from build123d import *

# Parameters (mm, degrees)
F0_R     = 160
F0_R_2   = 4.5
F0_R_3   = 4
F0_R_4   = 3.5
F0_R_5   = 125
F1_DEPTH = 5


with BuildPart() as f1:
    # F0 (on Top) → F1 (new body)
    with BuildSketch(Plane.XY):
        Circle(F0_R)
        with Locations((-89.58033, -123.296747)):
            Circle(F0_R_2, mode=Mode.SUBTRACT)
        with Locations((-123.296747, -89.58033)):
            Circle(F0_R_2, mode=Mode.SUBTRACT)
        with Locations((-106.988743, -92.985752)):
            Circle(F0_R_3, mode=Mode.SUBTRACT)
        with Locations((-91.955953, -96.538456)):
            Circle(F0_R_4, mode=Mode.SUBTRACT)
        with Locations((-47.095167, -144.944019)):
            Circle(F0_R_2, mode=Mode.SUBTRACT)
        with Locations((-73.121028, -121.182326)):
            Circle(F0_R_3, mode=Mode.SUBTRACT)
        with Locations((-32.197696, -137.533162)):
            Circle(F0_R_3, mode=Mode.SUBTRACT)
        with Locations((-17.947687, -131.571308)):
            Circle(F0_R_4, mode=Mode.SUBTRACT)
        with Locations((-57.726149, -119.915761)):
            Circle(F0_R_4, mode=Mode.SUBTRACT)
        with Locations((-144.944019, -47.095167)):
            Circle(F0_R_2, mode=Mode.SUBTRACT)
        with Locations((-130.485633, -55.703517)):
            Circle(F0_R_3, mode=Mode.SUBTRACT)
        with Locations((-117.286447, -63.727727)):
            Circle(F0_R_4, mode=Mode.SUBTRACT)
        with Locations((-131.238105, -24.695316)):
            Circle(F0_R_4, mode=Mode.SUBTRACT)
        with Locations((-141.31166, -12.985067)):
            Circle(F0_R_3, mode=Mode.SUBTRACT)
        with Locations((0, -152.403161)):
            Circle(F0_R_2, mode=Mode.SUBTRACT)
        with Locations((11.775392, -140.437726)):
            Circle(F0_R_3, mode=Mode.SUBTRACT)
        with Locations((23.485642, -130.364171)):
            Circle(F0_R_4, mode=Mode.SUBTRACT)
        with Locations((47.095167, -144.944019)):
            Circle(F0_R_2, mode=Mode.SUBTRACT)
        with Locations((54.493843, -129.611699)):
            Circle(F0_R_3, mode=Mode.SUBTRACT)
        with Locations((62.518052, -116.412512)):
            Circle(F0_R_4, mode=Mode.SUBTRACT)
        with Locations((89.58033, -123.296747)):
            Circle(F0_R_2, mode=Mode.SUBTRACT)
        with Locations((91.776078, -106.114808)):
            Circle(F0_R_3, mode=Mode.SUBTRACT)
        with Locations((95.328782, -91.082019)):
            Circle(F0_R_4, mode=Mode.SUBTRACT)
        with Locations((123.296747, -89.58033)):
            Circle(F0_R_2, mode=Mode.SUBTRACT)
        with Locations((119.972651, -72.247093)):
            Circle(F0_R_3, mode=Mode.SUBTRACT)
        with Locations((118.706086, -56.852215)):
            Circle(F0_R_4, mode=Mode.SUBTRACT)
        with Locations((144.944019, -47.095167)):
            Circle(F0_R_2, mode=Mode.SUBTRACT)
        with Locations((136.323487, -31.323761)):
            Circle(F0_R_3, mode=Mode.SUBTRACT)
        with Locations((130.361633, -17.073752)):
            Circle(F0_R_4, mode=Mode.SUBTRACT)
        with Locations((-152.403161, 0)):
            Circle(F0_R_2, mode=Mode.SUBTRACT)
        with Locations((-132.445243, 16.738012)):
            Circle(F0_R_4, mode=Mode.SUBTRACT)
        with Locations((-138.407097, 30.988021)):
            Circle(F0_R_3, mode=Mode.SUBTRACT)
        with Locations((-144.944019, 47.095167)):
            Circle(F0_R_2, mode=Mode.SUBTRACT)
        with Locations((-120.789696, 56.516474)):
            Circle(F0_R_4, mode=Mode.SUBTRACT)
        with Locations((-122.056261, 71.911353)):
            Circle(F0_R_3, mode=Mode.SUBTRACT)
        with Locations((-123.296747, 89.58033)):
            Circle(F0_R_2, mode=Mode.SUBTRACT)
        with Locations((-97.412391, 90.746279)):
            Circle(F0_R_4, mode=Mode.SUBTRACT)
        with Locations((-93.859687, 105.779068)):
            Circle(F0_R_3, mode=Mode.SUBTRACT)
        with Locations((-89.58033, 123.296747)):
            Circle(F0_R_2, mode=Mode.SUBTRACT)
        with Locations((-64.601662, 116.076772)):
            Circle(F0_R_4, mode=Mode.SUBTRACT)
        with Locations((-56.577452, 129.275959)):
            Circle(F0_R_3, mode=Mode.SUBTRACT)
        with Locations((-47.095167, 144.944019)):
            Circle(F0_R_2, mode=Mode.SUBTRACT)
        with Locations((-25.569251, 130.028431)):
            Circle(F0_R_4, mode=Mode.SUBTRACT)
        with Locations((-13.859001, 140.101986)):
            Circle(F0_R_3, mode=Mode.SUBTRACT)
        Circle(F0_R_5, mode=Mode.SUBTRACT)
        with Locations((139.228051, 12.649326)):
            Circle(F0_R_3, mode=Mode.SUBTRACT)
        with Locations((152.403161, 0)):
            Circle(F0_R_2, mode=Mode.SUBTRACT)
        with Locations((129.154496, 24.359576)):
            Circle(F0_R_4, mode=Mode.SUBTRACT)
        with Locations((115.202838, 63.391987)):
            Circle(F0_R_4, mode=Mode.SUBTRACT)
        with Locations((128.402024, 55.367777)):
            Circle(F0_R_3, mode=Mode.SUBTRACT)
        with Locations((144.944019, 47.095167)):
            Circle(F0_R_2, mode=Mode.SUBTRACT)
        with Locations((55.64254, 119.580021)):
            Circle(F0_R_4, mode=Mode.SUBTRACT)
        with Locations((15.864077, 131.235568)):
            Circle(F0_R_4, mode=Mode.SUBTRACT)
        with Locations((30.114086, 137.197422)):
            Circle(F0_R_3, mode=Mode.SUBTRACT)
        with Locations((0, 152.403161)):
            Circle(F0_R_2, mode=Mode.SUBTRACT)
        with Locations((71.037418, 120.846586)):
            Circle(F0_R_3, mode=Mode.SUBTRACT)
        with Locations((47.095167, 144.944019)):
            Circle(F0_R_2, mode=Mode.SUBTRACT)
        with Locations((89.872344, 96.202716)):
            Circle(F0_R_4, mode=Mode.SUBTRACT)
        with Locations((104.905133, 92.650012)):
            Circle(F0_R_3, mode=Mode.SUBTRACT)
        with Locations((123.296747, 89.58033)):
            Circle(F0_R_2, mode=Mode.SUBTRACT)
        with Locations((89.58033, 123.296747)):
            Circle(F0_R_2, mode=Mode.SUBTRACT)
    extrude(amount=F1_DEPTH)


solid = f1.part
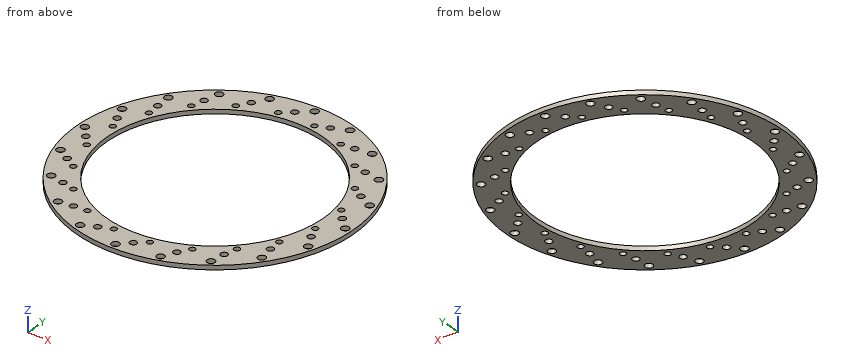
Here's how the part is built. I have some questions about the finished solid (model axes, mm). Round coordinates to 2 decimals unless told otherwise and drop trailing zeros. Loops run counter-clockwise (first coordinate to the right, second up) from the corner with the lowest first, then second, coordinate; pieces in that order, holes last. Notation, with made-up numbers: (32.5, 41) - (68.5, 41) arc R23 ccw to (68.5, 74) - close; hole circle Ø5 at (-4, 7). An arc over 180 degrees is marked (long way). One line per question, with ' | ' between items. Start each with the question number.
Q1. Will these pins go through, and if not, where does the flat tip stop? pin 1 (1 mm diameter, centred on y = -64.5, z = 2.5, fed in from -X); pin 2 (1 mm diameter, centred on y = -78, z = 4.5, fed in from -X); pin 3 (5 mm diameter, centred on x = -13.86, y = 140.1, fed in from -Z); pin 4 (1.5 mm diameter, centred on y = -83, z = 3.5, fed in from +X).
Q2. Please list where these lines run through material, in increasing order: line 1 (Y direction, x = -46, z = 3.25); line 2 (X direction, y = 129, z = 0.9); line 3 (Y direction, x = 70.5, z = 2.55). Write a range as [from, to].
Q3. I want a section at A-A (y = 0). Write out the boundary of the cut face in (x, z), then the cut area to 3 significant figures.
Q4. I want a section at C-C (z = 2.3). State how many separate pieces and enclosed holes the cut face has, then the cut area to 3 significant figures.
Response values:
1) pin 1: stops at x = -146.64 | pin 2: stops at x = -139.98 | pin 3: passes through | pin 4: stops at x = 137.24
2) line 1: y = [-153.24, -149.31], [-140.58, -116.23], [116.23, 140.58], [149.31, 153.24] | line 2: x = [-94.65, -60.57], [-52.59, -28.91], [-22.22, 13.17], [18.56, 94.65] | line 3: y = [-143.63, -103.22], [103.22, 116.88], [124.81, 143.63]
3) outline: (-160, 0) - (-156.9, 0) - (-156.9, 5) - (-160, 5) - close; (-147.9, 0) - (-125, 0) - (-125, 5) - (-147.9, 5) - close; (125, 0) - (147.9, 0) - (147.9, 5) - (125, 5) - close; (156.9, 0) - (160, 0) - (160, 5) - (156.9, 5) - close | area: 260 mm²
4) separate pieces: 1 | enclosed holes: 61 | area: 28,300 mm²
